Autodesk Inventor part; units mm, degrees
ref_plane "YZ Plane" through (0, 0, 0) normal (1, 0, 0) x (0, 1, 0)
ref_plane "XZ Plane" through (0, 0, 0) normal (0, 1, 0) x (-1, 0, 0)
ref_plane "XY Plane" through (0, 0, 0) normal (0, 0, 1) x (1, 0, 0)
sketch "スケッチ1" plane through (0, 0, 0) normal (0, 0, 1) x (1, 0, 0)
  circle A0 centre (0, 0) radius 4
  dimension "d0" = 8
extrude "押し出し1" add sketch "スケッチ1" along normal blind 8
sketch "スケッチ2" plane through (0, 0, 0) normal (0, 0, 1) x (1, 0, 0)
  line L0 (-6, -6) -> (6, -6)
  line L1 (6, -6) -> (6, 6)
  line L2 (6, 6) -> (-6, 6)
  line L3 (-6, 6) -> (-6, -6)
  line L4 (-6, -6) -> (6, 6) construction
  line L5 (6, -6) -> (-6, 6) construction
  point P0 (0, 0)
  dimension "d3" = 12
  dimension "d4" = 12
extrude "押し出し2" add sketch "スケッチ2" against normal blind 12.5
chamfer "面取り1" distance 2.1 angle 45 1 edges at (6, 6, -6.25)
chamfer "面取り2" distance 2.1 angle 45 1 edges at (-6, 6, -6.25)
chamfer "面取り3" distance 2.1 angle 45 1 edges at (-6, -6, -6.25)
chamfer "面取り4" distance 2.1 angle 45 1 edges at (6, -6, -6.25)
sketch "スケッチ3" plane through (0, 0, -12.5) normal (0, 0, -1) x (-1, 0, 0)
  circle A0 centre (0, 0) radius 5.5
  dimension "d19" = 11
extrude "押し出し3" add sketch "スケッチ3" along normal blind 38.75
sketch "スケッチ4" plane through (0, 0, -51.25) normal (0, 0, -1) x (-1, 0, 0)
  line L0 (5.875, 5.875) -> (-5.875, 5.875)
  line L1 (-5.875, 5.875) -> (-5.875, -5.875)
  line L2 (-5.875, -5.875) -> (5.875, -5.875)
  line L3 (5.875, -5.875) -> (5.875, 5.875)
  line L4 (5.875, 5.875) -> (-5.875, -5.875) construction
  line L5 (-5.875, 5.875) -> (5.875, -5.875) construction
  point P0 (0, 0)
  dimension "d22" = 11.75
  dimension "d23" = 11.75
extrude "押し出し4" add sketch "スケッチ4" along normal blind 10
chamfer "面取り5" distance 1.4 angle 45 1 edges at (-5.875, -5.875, -56.25)
chamfer "面取り6" distance 1.4 angle 45 1 edges at (-5.875, 5.875, -56.25)
chamfer "面取り7" distance 1.4 angle 45 1 edges at (5.875, -5.875, -56.25)
chamfer "面取り8" distance 1.4 angle 45 1 edges at (5.875, 5.875, -56.25)
sketch "スケッチ5" plane through (3.9, 6, 0) normal (0, 1, 0) x (1, 0, 0)
  circle A0 centre (-3.9, 8) radius 2
  point P0 (-3.9, 0)
  dimension "d38" = 4
  dimension "d39" = 8
extrude "押し出し5" cut sketch "スケッチ5" against normal blind 10
sketch "スケッチ6" plane through (-4.475, 5.875, -51.25) normal (0, 1, 0) x (1, 0, 0)
  circle A0 centre (4.475, 5) radius 2
  line L0 (0, 0) -> (8.95, 0)
  point P0 (4.475, -51.25)
  dimension "d42" = 4
  dimension "d43" = 5
extrude "押し出し6" cut sketch "スケッチ6" against normal blind 10
sketch "スケッチ7" plane through (0, 0, 8) normal (0, 0, 1) x (1, 0, 0)
  circle A0 centre (0, 0) radius 2.25
  dimension "d46" = 4.5
extrude "押し出し7" cut sketch "スケッチ7" against normal blind 40
properties part number "air_cylinder_15_part1_sa" material "アルミニウム 6061-AHC"
Geometry: final body of the model. Coordinates: model frame, mm. A direction names the side the tool comes from. Round coordinates to 2 decimals unless told otherwise and drop trailing zeros. Loops run counter-clockwise (first coordinate to the right, second up) from the corner with the lowest first, then second, coordinate; pieces in that order, holes last. Notation, with made-up numbers: M 40,-39 L 91,-39 A30 cw 91,-11 Z; hole C -16,-7.75 d4. An arc over 180 degrees is marked long. Put each result on its own line as item: value. Start each with the question number.
(1) Contact query for flat-ended pins moving along their axis: pin 1 Ø3.5 at (x, z) = (0, -56.25) entering from -Y (3 decimals); pin 2 Ø3.5 at (x, z) = (0, -8) entering from +Y; pin 3 Ø5 at (x, z) = (2.5, -14) entering from -Y; pin 4 Ø4.5 at (x, z) = (-0.5, -56) entering from +Y (3 decimals). Output: stop coordinate, or through.
(2) Section query C-C (z = -56.25). Return loops of the section in (x, y) (3 decimals).
(3) Section query A-A (y = 0). Return loops of the section in (x, z) (3 decimals), then the cut area to 3 significant figures.
(4) Section query D-D (x = -3). Return loops of the section in (y, z) (3 decimals), then the cut area to 3 significant figures.
(5) Set-up query: faces 1 (the face through (0, -5.875, -56)), 2 (the face through (1.19, 5.37, -31.6)), 3 (the face through (5, -4.9, -6.2)), 4 (the face through (-1.4, 4.1, 0)). Return all of +Z, -Z, +X, -X, +Y, -Y with unobstructed straight access to the full face (end or side cutting, diameter ignored); none if empty.
(6) Draft query along X for faces 5 (the face through (5.17, 5.18, -56.18)), 6 (the face through (2.146, 0.676, -11.72)), 7 (the face through (0, 0, -32)), 8 (the face through (2, -2, 8)). Return one class per face: +X half, -X half, draft (parallel to the pull), parting line (faces both ways), or undercut.
(7) Material intervals for line 1 along Z through (x, y) = (0, 2.5); line 2 along Z through (x, y) = (-3.5, 5.5); line 3 along Y through (x, z) = (0.25, -3), sorted ascending. Write a range as [from, to].
Findings below:
1. pin 1: stops at y = -5.875
1. pin 2: stops at y = -4
1. pin 3: stops at y = -6
1. pin 4: stops at y = 5.875
2. outline: M -5.875,-4.475 L -4.475,-5.875 L 4.475,-5.875 L 5.875,-4.475 L 5.875,4.475 L 4.475,5.875 L 2,5.875 L 2,-4.125 L -2,-4.125 L -2,5.875 L -4.475,5.875 L -5.875,4.475 Z
3. outline: M -6,-12.5 L -5.5,-12.5 L -5.5,-51.25 L -5.875,-51.25 L -5.875,-61.25 L 5.875,-61.25 L 5.875,-51.25 L 5.5,-51.25 L 5.5,-12.5 L 6,-12.5 L 6,0 L 4,0 L 4,8 L 2.25,8 L 2.25,-32 L -2.25,-32 L -2.25,8 L -4,8 L -4,0 L -6,0 Z; hole C 0,-56.25 d4
3. area: 565 mm2
4. outline: M -6,-12.5 L -4.61,-12.5 L -4.61,-51.25 L -5.875,-51.25 L -5.875,-61.25 L 5.875,-61.25 L 5.875,-51.25 L 4.61,-51.25 L 4.61,-12.5 L 6,-12.5 L 6,0 L 2.646,0 L 2.646,8 L -2.646,8 L -2.646,0 L -6,0 Z
4. area: 667 mm2
5. face 1: -Z, +X, -X, -Y
5. face 2: none
5. face 3: +Z, +X, -Y
5. face 4: +Z
6. face 5: +X half
6. face 6: undercut
6. face 7: undercut
6. face 8: draft
7. line 1: z = [-61.25, -58.25], [-54.25, -10], [-6, 8]
7. line 2: z = [-61.25, -51.25], [-12.5, 0]
7. line 3: y = [-6, -2.24], [2.24, 6]
